from build123d import *

# Parameters (mm, degrees)
BOSS_EXTRUDE1_DEPTH = 200
CUT_EXTRUDE1_DEPTH  = 466.401952215
FILLET1_R           = 10
BOSS_EXTRUDE2_DEPTH = 12


with BuildPart() as part:
    # Sketch1 → Boss-Extrude1 (new body)
    with BuildSketch(Plane.XY):
        Polygon((0, 0), (360, 0), (360, -20), (400, -20), (400, 118), (222.295517328, 220.597730907), (185, 156), (185, 38), (0, 38), align=None)
    extrude(amount=BOSS_EXTRUDE1_DEPTH)

    # Sketch2 → Cut-Extrude1 (cut, through all)
    with BuildSketch(Plane(origin=(71.200018505, -41.10734985, 0), x_dir=(0, 0, 1), z_dir=(-0.8660254037844399, 0.4999999999999977, 0))):
        Polygon((30, 272.190997647), (170, 272.190997647), (150, 302.190997647), (50, 302.190997647), align=None)
    extrude(amount=-CUT_EXTRUDE1_DEPTH, mode=Mode.SUBTRACT)

    # Fillet1
    fillet1_edges = [part.edges().sort_by_distance(p)[0] for p in [
        (0, 19, 0),
        (0, 19, 200),
    ]]
    fillet(fillet1_edges, radius=FILLET1_R)

    # Sketch3 → Boss-Extrude2 (add)
    with BuildSketch(Plane(origin=(0, 38, 0), x_dir=(1, 0, 0), z_dir=(0, 1, 0))):
        with BuildLine():
            Line((50, -135), (50, -65))
            ThreePointArc((50, -65), (87.999995632, -26.999991264), (126, -64.999991264))
            Line((126, -64.999991264), (126, -135))
            ThreePointArc((126, -135), (88, -173), (50, -135))
        make_face()
        with BuildLine():
            Line((68.5, -135), (68.5, -65))
            ThreePointArc((68.5, -65), (87.999995632, -45.499991264), (107.5, -64.999991264))
            Line((107.5, -64.999991264), (107.5, -135))
            ThreePointArc((107.5, -135), (88, -154.5), (68.5, -135))
        make_face(mode=Mode.SUBTRACT)
    extrude(amount=BOSS_EXTRUDE2_DEPTH)


solid = part.part
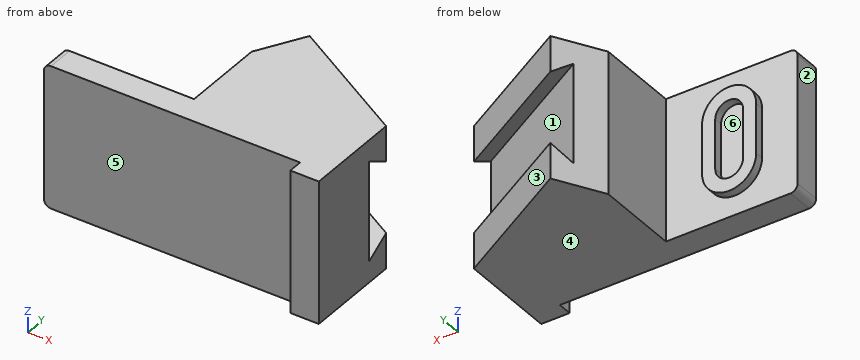
Build history of the part. All positions in model axes, mm. Face numbers are marked on the shaded views. A direction names the side the tool comes from. Coordinates: 2 decimals unless noted, no trailing zeros. Write each loop counter-clockwise with the first axis right and the second up, starting at its lowest first coordinate (ties: lowest second). Pieces come first, ordered by that corner, then holes.
(1) 3-axis set-ups, long thin cutter, end or side, ignore diameter. For the marked faces 4, 5 and 6: which of +Z, -Z, +X, -X, +Y, -Y reach the whole face in a straight line?
(2) Mould opens along Y. For the marked faces 1, 2 and 3 say: pulls with the +Y half, pulls with the -Y half, needs draft (parallel to the pull), parting line crosses it, or undercut.
(3) Cut at B-B on y = 206. List the corners of the cut face in (x, z).
(4) Pin check, flat tips, straight feed: pin 1 Ø19.5 at (x, z) = (97, 125.5) entering from +Y; pin 2 Ø23 at (x, z) = (105.5, 123) entering from +Y; pin 3 Ø1.5 at (y, z) = (158, 61) entering from -X. Stop position of each tip, or through.
(5) Cut at D-D on y = 65. List the corners of the cut face in (x, z), and give its area (3 significant figures).
(6) Cut at C-C on x = 88. List the corners of the cut face in (y, z), and give its area (3 significant figures).
(7) Drill centre lines: line 1 (X direction, y = 45.5, z = 122); line 2 (Y direction, x = 173, z = 157); line 3 (Y direction, x = 383, z = 44.5). Where is each one in solid material? Low to high.
(8) Cut at A-A on z = 99.5. List the corners of the cut face in (x, y).
Working result:
1. face 4: -Z, +X, -X, +Y, -Y
1. face 5: +Z, -Z, -X, -Y
1. face 6: +Y
2. face 1: undercut
2. face 2: needs draft
2. face 3: pulls with the +Y half
3. outline: (213.87, 0) - (247.58, 0) - (247.58, 50) - (213.87, 38.76) - close; (213.87, 161.24) - (247.58, 150) - (247.58, 200) - (213.87, 200) - close
4. pin 1: stops at y = 38
4. pin 2: stops at y = 50
4. pin 3: stops at x = 185.72
5. outline: (185, 0) - (400, 0) - (400, 200) - (185, 200) - close
5. area: 43,000 mm2
6. outline: (0, 0) - (38, 0) - (38, 27) - (50, 27) - (50, 45.5) - (38, 45.5) - (38, 154.5) - (50, 154.5) - (50, 173) - (38, 173) - (38, 200) - (0, 200) - close
6. area: 8,040 mm2
7. line 1: x = 50 to 68.5, 107.5 to 126, 185 to 400
7. line 2: y = 0 to 38
7. line 3: y = -20 to 93.17, 118.29 to 127.81
8. outline: (0, 0) - (360, 0) - (360, -20) - (400, -20) - (400, 83.36) - (207.3, 194.62) - (185, 156) - (185, 38) - (126, 38) - (126, 50) - (107.5, 50) - (107.5, 38) - (68.5, 38) - (68.5, 50) - (50, 50) - (50, 38) - (0, 38) - close
